```python
from build123d import *

# Parameters (mm, degrees)
SKETCH1_R           = 15.875
BOSS_EXTRUDE1_DEPTH = 42.8625
SKETCH2_R           = 17.4625
BOSS_EXTRUDE2_DEPTH = 17.4625
SKETCH3_R           = 6.35
BOSS_EXTRUDE3_DEPTH = 1.5875
SKETCH4_R           = 2.38125
BOSS_EXTRUDE4_DEPTH = 11.1125
CUT_EXTRUDE1_START  = -9.525
CUT_EXTRUDE1_DEPTH  = 9.525
SKETCH6_R           = 4.7625
BOSS_EXTRUDE5_DEPTH = 1.5875


with BuildPart() as part:
    # Sketch1 → Boss-Extrude1 (new body)
    with BuildSketch(Plane(origin=(0, 0, 0), x_dir=(1, 0, 0), z_dir=(0, 1, 0))):
        with Locations(Location((0, 0, 0), (0, 0, 270))):
            Circle(SKETCH1_R)
    extrude(amount=BOSS_EXTRUDE1_DEPTH)

    # Sketch2 → Boss-Extrude2 (add)
    with BuildSketch(Plane(origin=(0, 42.8625, 0), x_dir=(1, 0, 0), z_dir=(0, 1, 0))):
        with Locations(Location((0, 0, 0), (0, 0, 270))):
            Circle(SKETCH2_R)
    extrude(amount=BOSS_EXTRUDE2_DEPTH)

    # Sketch3 → Boss-Extrude3 (add)
    with BuildSketch(Plane(origin=(0, 60.325, 0), x_dir=(1, 0, 0), z_dir=(0, 1, 0))):
        with Locations(Location((0, -8.73252, 0), (0, 0, 270))):
            Circle(SKETCH3_R)
    extrude(amount=BOSS_EXTRUDE3_DEPTH)

    # Sketch4 → Boss-Extrude4 (add)
    with BuildSketch(Plane(origin=(0, 61.9125, 0), x_dir=(1, 0, 0), z_dir=(0, 1, 0))):
        with Locations(Location((0, -8.73252, 0), (0, 0, 270))):
            Circle(SKETCH4_R)
    extrude(amount=BOSS_EXTRUDE4_DEPTH)

    # Sketch5 → Cut-Extrude1 (cut)
    with BuildSketch(Plane(origin=(0, 73.025, 0), x_dir=(1, 0, 0), z_dir=(0, 1, 0)).offset(CUT_EXTRUDE1_START)):
        with BuildLine():
            Line((-2.062222993, -7.541895), (2.062222993, -7.541895))
            ThreePointArc((2.062222993, -7.541895), (0, -6.35127), (-2.062222993, -7.541895))
        make_face()
    extrude(amount=CUT_EXTRUDE1_DEPTH, mode=Mode.SUBTRACT)

    # Sketch6 → Boss-Extrude5 (add)
    with BuildSketch(Plane.XZ):
        with Locations(Location((0, 0, 0), (0, 0, 90))):
            Circle(SKETCH6_R)
    extrude(amount=BOSS_EXTRUDE5_DEPTH)


solid = part.part
```
Build history of the part. All positions in model axes, mm. A direction names the side the tool comes from. Give positions to 0.01 mm unless a question says otherwise; leave off trailing zeros. Loops run counter-clockwise (first coordinate to the right, second up) from the corner with the lowest first, then second, coordinate; pieces in that order, holes last. Notation, with made-up numbers: (76, -37) - (118, -37) arc R20 ccw to (118, -17) - close; hole circle Ø8 at (41, 12.25). An arc over 180 degrees is marked (long way). Use a Markdown table: item, result.
(1) Band-saw the part on B-B (x = 0). Give the cut face in (y, z) (1 decimal), and give its area (3 significant figures).
Taken from the geometry:
| item | result |
|---|---|
| outline | (-1.6, -4.8) - (0, -4.8) - (0, -15.9) - (42.9, -15.9) - (42.9, -17.5) - (60.3, -17.5) - (60.3, 2.4) - (61.9, 2.4) - (61.9, 6.4) - (63.5, 6.4) - (63.5, 7.5) - (73, 7.5) - (73, 11.1) - (61.9, 11.1) - (61.9, 15.1) - (60.3, 15.1) - (60.3, 17.5) - (42.9, 17.5) - (42.9, 15.9) - (0, 15.9) - (0, 4.8) - (-1.6, 4.8) - close |
| area | 2,050 mm2 |
(2) Drop flat-ended pins along their axis: pin 1 Ø3.5 at (x, y) = (1, 69.5) entering from -Z; pin 2 Ø8 at (x, y) = (-13.5, 9) entering from -Z; pin 3 Ø5 at (x, z) = (-11, 11) entering from +Y (3 decimals). Give the stop position or say it passes through.
Taken from the geometry:
| item | result |
|---|---|
| pin 1 | z = 7.54 |
| pin 2 | z = -12.72 |
| pin 3 | y = 60.325 |
(3) Band-saw the part on C-C (y = 41). Give the cut face in (x, z) (3 decimals), and give its area (3 significant figures).
Taken from the geometry:
| item | result |
|---|---|
| outline | circle Ø31.75 at (0, 0) |
| area | 792 mm2 |
(4) Wall check: line 1 along Y through (x, z) = (15, -3) (3 decimals); line 2 along Y through (x, z) = (7, -14.5) (1 decimal); line 3 along X through (y, z) = (8.5, -7). Give the ranges that are in metal, low to high.
Taken from the geometry:
| item | result |
|---|---|
| line 1 | 0 to 60.325 |
| line 2 | 42.9 to 60.3 |
| line 3 | -14.25 to 14.25 |
(5) Band-saw the part on D-D (z = -9). Give the cut face in (x, y) (1 decimal), and give its area (3 significant figures).
Taken from the geometry:
| item | result |
|---|---|
| outline | (-15, 42.9) - (-13.1, 42.9) - (-13.1, 0) - (13.1, 0) - (13.1, 42.9) - (15, 42.9) - (15, 60.3) - (-15, 60.3) - close |
| area | 1,640 mm2 |
(6) Which spindle directions (+Z, -Z, +X, -X, +Y, -Y) get a long thin tool onto all of the face, cutting with end or side? Do faces 1 (the face through (0.1, 61.912, 11.5)), 2 (the face through (-3, 0, -4)), 3 (the face through (0, 68, 7.542)). Say none if no direction does.
Taken from the geometry:
| item | result |
|---|---|
| face 1 | +Y |
| face 2 | -Y |
| face 3 | -Z, +X, -X, +Y |
(7) Band-saw the part on A-A (z = 0). Give the cut face in (x, y) (1 decimal).
Taken from the geometry:
| item | result |
|---|---|
| outline | (-17.5, 42.9) - (-15.9, 42.9) - (-15.9, 0) - (-4.8, 0) - (-4.8, -1.6) - (4.8, -1.6) - (4.8, 0) - (15.9, 0) - (15.9, 42.9) - (17.5, 42.9) - (17.5, 60.3) - (-17.5, 60.3) - close |
